from build123d import *

# Parameters (mm, degrees)
SKETCH1_W                                    = 406.4
SKETCH1_H                                    = 152.4
BOSS_EXTRUDE1_DEPTH                          = 12
CUT_EXTRUDE1_DEPTH                           = 12
BOSS_EXTRUDE2_REACH                          = 249.278
SKETCH4_R                                    = 19.49375
SKETCH4_R_2                                  = 13.49375
BOSS_EXTRUDE3_DEPTH                          = 50
SKETCH4_2_R                                  = 13.49375
CUT_EXTRUDE2_DEPTH                           = 50
SKETCH4_3_R                                  = 13.49375
BOSS_EXTRUDE4_DEPTH                          = 12
MIRROR1_AT_THE_SECOND_PLANE_COPY_1_SKETC_R   = 19.49375
MIRROR1_AT_THE_SECOND_PLANE_COPY_1_SKETC_R_2 = 13.49375
MIRROR1_AT_THE_SECOND_PLANE_COPY_1_DEPTH     = 50
MIRROR1_AT_THE_SECOND_PLANE_COPY_2_SKETC_R   = 13.49375
MIRROR1_AT_THE_SECOND_PLANE_COPY_2_DEPTH     = 50
MIRROR1_AT_THE_SECOND_PLANE_COPY_3_SKETC_R   = 13.49375
MIRROR1_AT_THE_SECOND_PLANE_COPY_3_DEPTH     = 12


with BuildPart() as part:
    # Sketch1 → Boss-Extrude1 (new body)
    with BuildSketch(Plane(origin=(0, 0, 0), x_dir=(1, 0, 0), z_dir=(0, 1, 0))):
        Rectangle(SKETCH1_W, SKETCH1_H)
    extrude(amount=BOSS_EXTRUDE1_DEPTH)

    # Sketch2 → Cut-Extrude1 (cut)
    with BuildSketch(Plane(origin=(0, 12, 0), x_dir=(1, 0, 0), z_dir=(0, 1, 0))):
        Polygon((-203.2, -64.2), (-191.2, -64.2), (191.2, -64.2), (191.2, 64.2), (-191.2, 64.2), (-203.2, 64.2), align=None)
    extrude(amount=-CUT_EXTRUDE1_DEPTH, mode=Mode.SUBTRACT)

    # Sketch3 → Boss-Extrude2 (add, up to next)
    with BuildSketch(Plane.XY.offset(-64.2), mode=Mode.PRIVATE) as boss_extrude2_sk1:
        Polygon((-191.2, 0), (191.2, 12), (191.2, 0), align=None)
    boss_extrude2_tool1 = extrude(boss_extrude2_sk1.sketch, amount=BOSS_EXTRUDE2_REACH, mode=Mode.PRIVATE) - part.part
    add(boss_extrude2_tool1.solids().sort_by_distance((63.733333, 4, -64.2))[0])

    # Sketch4 → Boss-Extrude3 (add)
    with BuildSketch(Plane(origin=(0, 0, 0), x_dir=(1, 0, 0), z_dir=(0, 1, 0))):
        with Locations(Location((-203.2, -76.2, 0), (0, 0, 52.005784389))):
            Circle(SKETCH4_R)
        with Locations(Location((-203.2, -76.2, 0), (0, 0, 62.785492025))):
            Circle(SKETCH4_R_2, mode=Mode.SUBTRACT)
    boss_extrude3 = extrude(amount=BOSS_EXTRUDE3_DEPTH)

    # Sketch4_2 → Cut-Extrude2 (cut)
    with BuildSketch(Plane(origin=(0, 0, 0), x_dir=(1, 0, 0), z_dir=(0, 1, 0))):
        with Locations(Location((-203.2, -76.2, 0), (0, 0, 270))):
            Circle(SKETCH4_2_R)
    cut_extrude2 = extrude(amount=CUT_EXTRUDE2_DEPTH, mode=Mode.SUBTRACT)

    # Sketch4_3 → Boss-Extrude4 (add)
    with BuildSketch(Plane(origin=(0, 0, 0), x_dir=(1, 0, 0), z_dir=(0, 1, 0))):
        with Locations(Location((-203.2, -76.2, 0), (0, 0, 270))):
            Circle(SKETCH4_3_R)
    boss_extrude4 = extrude(amount=BOSS_EXTRUDE4_DEPTH)

    # Mirror1: Boss-Extrude3, Cut-Extrude2, Boss-Extrude4 across plane
    add(boss_extrude3.mirror(Plane(origin=(0, 0, 0), x_dir=(0, 0, 1), z_dir=(1, 0, 0))))
    add(cut_extrude2.mirror(Plane(origin=(0, 0, 0), x_dir=(0, 0, 1), z_dir=(1, 0, 0))), mode=Mode.SUBTRACT)
    add(boss_extrude4.mirror(Plane(origin=(0, 0, 0), x_dir=(0, 0, 1), z_dir=(1, 0, 0))))

    # Mirror1 at the second plane: Boss-Extrude3, Cut-Extrude2, Boss-Extrude4 across plane
    add(boss_extrude3.mirror(Plane.XY))
    add(cut_extrude2.mirror(Plane.XY), mode=Mode.SUBTRACT)
    add(boss_extrude4.mirror(Plane.XY))

    # Mirror1 at the second plane copy 1 sketc → Mirror1 at the second plane copy 1 (add)
    with BuildSketch(Plane(origin=(0, 0, 0), x_dir=(-1, 0, 0), z_dir=(0, 1, 0))):
        with Locations(Location((-203.2, -76.2, 0), (0, 0, 52.005784389))):
            Circle(MIRROR1_AT_THE_SECOND_PLANE_COPY_1_SKETC_R)
        with Locations(Location((-203.2, -76.2, 0), (0, 0, 62.785492025))):
            Circle(MIRROR1_AT_THE_SECOND_PLANE_COPY_1_SKETC_R_2, mode=Mode.SUBTRACT)
    extrude(amount=MIRROR1_AT_THE_SECOND_PLANE_COPY_1_DEPTH)

    # Mirror1 at the second plane copy 2 sketc → Mirror1 at the second plane copy 2 (cut)
    with BuildSketch(Plane(origin=(0, 0, 0), x_dir=(-1, 0, 0), z_dir=(0, 1, 0))):
        with Locations(Location((-203.2, -76.2, 0), (0, 0, 270))):
            Circle(MIRROR1_AT_THE_SECOND_PLANE_COPY_2_SKETC_R)
    extrude(amount=MIRROR1_AT_THE_SECOND_PLANE_COPY_2_DEPTH, mode=Mode.SUBTRACT)

    # Mirror1 at the second plane copy 3 sketc → Mirror1 at the second plane copy 3 (add)
    with BuildSketch(Plane(origin=(0, 0, 0), x_dir=(-1, 0, 0), z_dir=(0, 1, 0))):
        with Locations(Location((-203.2, -76.2, 0), (0, 0, 270))):
            Circle(MIRROR1_AT_THE_SECOND_PLANE_COPY_3_SKETC_R)
    extrude(amount=MIRROR1_AT_THE_SECOND_PLANE_COPY_3_DEPTH)


solid = part.part
Build history of the part. All positions in model axes, mm. A direction names the side the tool comes from. Round coordinates to 2 decimals unless told otherwise and drop trailing zeros. Loops run counter-clockwise (first coordinate to the right, second up) from the corner with the lowest first, then second, coordinate; pieces in that order, holes last. Notation, with made-up numbers: (2, 52.5) -> (42, 52.5) arc R30 ccw to (42, 75.5) -> close; hole circle Ø1 at (-7.5, 54). An arc over 180 degrees is marked (long way). Use CSV: the item, a comma, the result in double quotes. Start each with the question number.
Q1. Saw through at D-D on x = 93.5. Give the cut face in (y, z).
Q2. Drill centre lines: L1, parallel to Z at x = 203.2, y = 39; L2, parallel to X at y = 20, z = 76.2; L3, parallel to X at y = 19.5, z = 84.5. Where is each one in solid material? Low to high.
Q3. Saw through at B-B on y = 30.5. Give the cut face in (x, z), and give its area (3 significant figures).
Q4. Saw through at A-A on x = -203.2. Give the cut face in (y, z), and give its area (3 significant figures).
Q5. Saw through at C-C on z = 9. Give the cut face in (x, y).
Q6. Which spindle directions (+Z, -Z, +X, -X, +Y, -Y) get a long thin tool onto all of the face, cutting with end or side? Do faces 1 (the face through (-3, 6, 76.2)), 2 (the face through (-3, 6, -76.2)), 3 (the face through (-203, 12, -76)), 4 (the face through (-199, 50, 63)). Say none if no direction does.
Q7. Flat gauge pins, fed straight in: pin 1 Ø6 at (x, z) = (196, 27) entering from +Y; pin 2 Ø1 at (y, z) = (12, -73) entering from -X; pin 3 Ø13 at (y, z) = (7, 20.5) entering from +X; pin 4 Ø12 at (x, y) = (-141.5, 20.5) entering from -Z. Where does each tip first touch, or does it go through?
Q8. Mould opens along X. For faces 5 (the face through (215.864, 24.65, 91.02)), 6 (the face through (203.2, 6, 1)), 7 (the face through (-3, 0, 1)) say: +X half, -X half, draft (parallel to the pull), parting line (faces both ways), or undercut.
Solutions:
1,outline,"(0, -76.2) -> (12, -76.2) -> (12, -64.2) -> (8.93, -64.2) -> (8.93, 64.2) -> (12, 64.2) -> (12, 76.2) -> (0, 76.2) -> close"
2,L1,"z = -95.69 to -89.69, -62.71 to -56.71, 56.71 to 62.71, 89.69 to 95.69"
2,L2,"x = -222.69 to -216.69, -189.71 to -183.71, 183.71 to 189.71, 216.69 to 222.69"
2,L3,"x = -220.84 to -213.84, -192.56 to -185.56, 185.56 to 192.56, 213.84 to 220.84"
3,outline,"circle Ø38.99 at (-203.2, -76.2); circle Ø38.99 at (-203.2, 76.2); circle Ø38.99 at (203.2, -76.2); circle Ø38.99 at (203.2, 76.2); hole circle Ø26.99 at (-203.2, -76.2); hole circle Ø26.99 at (-203.2, 76.2); hole circle Ø26.99 at (203.2, -76.2); hole circle Ø26.99 at (203.2, 76.2)"
3,area,"2,490 mm^2"
4,outline,"(0, -95.69) -> (50, -95.69) -> (50, -89.69) -> (12, -89.69) -> (12, -62.71) -> (50, -62.71) -> (50, -56.71) -> (0, -56.71) -> close; (0, 56.71) -> (50, 56.71) -> (50, 62.71) -> (12, 62.71) -> (12, 89.69) -> (50, 89.69) -> (50, 95.69) -> (0, 95.69) -> close"
4,area,"1,850 mm^2"
5,outline,"(-191.2, 0) -> (203.2, 0) -> (203.2, 12) -> (191.2, 12) -> close"
6,face 1,"+Z, +Y, -Y"
6,face 2,"-Z, +Y, -Y"
6,face 3,"+Y"
6,face 4,"+Z, -Z, +X, -X, +Y"
7,pin 1,"stops at y = 12"
7,pin 2,"stops at x = -222.51"
7,pin 3,"stops at x = 203.2"
7,pin 4,"passes through"
8,face 5,"undercut"
8,face 6,"+X half"
8,face 7,"draft"
